Autodesk Inventor part; units mm, degrees
ref_plane "YZ Plane" through (0, 0, 0) normal (1, 0, 0) x (0, 1, 0)
ref_plane "XZ Plane" through (0, 0, 0) normal (0, 1, 0) x (-1, 0, 0)
ref_plane "XY Plane" through (0, 0, 0) normal (0, 0, 1) x (1, 0, 0)
sketch "草图1" plane through (0, 0, 0) normal (0, 0, 1) x (1, 0, 0)
  arc A0 (7.5, 0) -> (-7.5, 0) centre (0, 0) ccw
  arc A1 (15, 0) -> (-15, 0) centre (0, 0) ccw
  line L0 (25, 5) -> (25, 0)
  line L1 (-25, 0) -> (-25, 5)
  line L2 (25, 0) -> (7.5, 0)
  line L3 (-7.5, 0) -> (-25, 0)
  line L4 (-25, 5) -> (-5.5902, 5)
  line L5 (5.5902, 5) -> (25, 5)
  line L6 (0, 0) -> (0, -4.0409)
  line L7 (0, 0) -> (2.0046, 0)
  arc A2 (5.5902, 5) -> (-5.5902, 5) centre (0, 0) ccw
  arc A3 (14.1421, 5) -> (-14.1421, 5) centre (0, 0) ccw
  dimension "d0" = 15
  dimension "d1" = 30
  dimension "d2" = 5
  dimension "d3" = 50
  dimension "d4" = 4.0409
  dimension "d5" = 2.0046
extrude "拉伸1" add sketch "草图1" along normal blind 40
sketch "草图2" plane through (0, 0, 40) normal (0, 0, 1) x (1, 0, 0)
  line L0 (14.1421, 5) -> (25, 5)
  line L1 (25, 5) -> (14.1421, 5)
  line L2 (25, 5) -> (25, 0)
  line L3 (25, 0) -> (15, 0)
  line L4 (7.5, 0) -> (25, 0)
  line L5 (-14.1421, 5) -> (-25, 5)
  line L6 (-14.1421, 5) -> (-25, 5)
  line L7 (-25, 5) -> (-25, 0)
  line L8 (-25, 0) -> (-15, 0)
  arc A0 (15, 0) -> (14.1421, 5) centre (0, 0) ccw
  arc A1 (-14.1421, 5) -> (-15, 0) centre (0, 0) ccw
extrude "拉伸2" cut sketch "草图2" against normal blind 5
pattern_linear "矩形阵列1" count 2 spacing 35 along (0, 0, -1) of "拉伸2"
fillet "圆角1" radius 0.25 2 edges at (14.1421, 5, 20) (-14.1421, 5, 20)
sketch "草图3" plane through (25, 5, 35) normal (0, 1, 0) x (1, 0, 0)
  circle A0 centre (-5, 25) radius 2.5
  circle A1 centre (-5, 5) radius 2.5
  circle A2 centre (-45, 25) radius 2.5
  circle A3 centre (-45, 5) radius 2.5
  line L0 (0, 30) -> (0, 0)
  line L1 (0, 30) -> (-10.6822, 30)
  line L2 (-10.6822, 0) -> (0, 0)
  line L3 (-50, 30) -> (-50, 0)
  line L4 (-50, 0) -> (-39.3178, 0)
  line L5 (-39.3178, 30) -> (-50, 30)
  point P0 (-25, 35)
  dimension "d14" = 5
  dimension "d15" = 5
  dimension "d16" = 5
  dimension "d17" = 5
  dimension "d18" = 5
  dimension "d19" = 5
  dimension "d20" = 5
  dimension "d21" = 5
  dimension "d22" = 5
  dimension "d23" = 5
  dimension "d24" = 5
  dimension "d25" = 5
extrude "拉伸3" cut sketch "草图3" against normal through all
properties part number "砂轮架带动曲柄轴盖"
Can you work these out from the model? Positions are in its coordinate system, mm. A direction names the side the tool comes from. Round coordinates to 2 decimals unless told otherwise and drop trailing zeros. Write each loop counter-clockwise with the first axis right and the second up, starting at its lowest first coordinate (ties: lowest second). Pieces come first, ordered by that corner, then holes. Notation, with made-up numbers: M -9,22.5 L 34,22.5 A21 ccw 34,28.5 Z; hole C 84.5,-38.5 d8. An arc over 180 degrees is marked long. Use a Markdown table: item, result.
Item 1: Which directions (+Z, -Z, +X, -X, +Y, -Y) give clear straight access to the entire face, cutting with the end or side of a thin tool? Please do faces 1 (the face through (-14.78, 2.57, 2.54)), 2 (the face through (-20, 5, 20)), 3 (the face through (20, 5, 20)).
Found:
| item | result |
|---|---|
| face 1 | -Z, -X, +Y |
| face 2 | +Z, -Z, -X, +Y |
| face 3 | +Z, -Z, +X, +Y |
Item 2: We'd pull the mould along Z, two halves only. Please class faces 4 (the face through (25, 3, 20)), 5 (the face through (-20, 3, 5)), 6 (the face through (-21.84, 2.54, 28.31)): released by +Z, released by -Z, zero draft, split by the parting line, or undercut.
Found:
| item | result |
|---|---|
| face 4 | zero draft |
| face 5 | released by -Z |
| face 6 | undercut |
Item 3: For pin 1 Ø3 at (x, z) = (-17.5, 25.5) entering from +Y; pin 2 Ø4 at (x, z) = (-20, 10) entering from +Y; pin 3 Ø5.5 at (x, y) = (-21, 3) entering from +Z; pin 4 Ø8 at (x, z) = (-9.5, 22) entering from +Y, each with a flat end and sliding along its axis, tell me the tip position at first contact or that it passes through.
Found:
| item | result |
|---|---|
| pin 1 | stops at y = 5 |
| pin 2 | passes through |
| pin 3 | stops at z = 35 |
| pin 4 | stops at y = 13.96 |
Item 4: I want a section at D-D (z = 26). List the corners of the cut face in (x, y) for me.
Found:
| item | result |
|---|---|
| outline | M -25,0 L -7.5,0 A7.5 cw 7.5,0 L 25,0 L 25,5 L 14.32,5 A0.25 cw 14.08,5.16 A15 ccw -14.08,5.16 A0.25 cw -14.32,5 L -25,5 Z |
Item 5: I want a section at C-C (y = 6.5). List the corners of the cut face in (x, z) for me.
Found:
| item | result |
|---|---|
| outline | M -13.52,0 L -3.74,0 L -3.74,40 L -13.52,40 Z; M 3.74,0 L 13.52,0 L 13.52,40 L 3.74,40 Z |
Item 6: I want a section at B-B (z = 8.5). List the corners of the cut face in (x, y) for me.
Found:
| item | result |
|---|---|
| outline | M -25,0 L -22,0 L -22,5 L -25,5 Z; M -18,0 L -7.5,0 A7.5 cw 7.5,0 L 18,0 L 18,5 L 14.32,5 A0.25 cw 14.08,5.16 A15 ccw -14.08,5.16 A0.25 cw -14.32,5 L -18,5 Z; M 22,0 L 25,0 L 25,5 L 22,5 Z |
Item 7: I want a section at A-A (x = 20). List the corners of the cut face in (y, z) for me, and give its area (3 significant figures).
Found:
| item | result |
|---|---|
| outline | M 0,5 L 5,5 L 5,7.5 L 0,7.5 Z; M 0,12.5 L 5,12.5 L 5,27.5 L 0,27.5 Z; M 0,32.5 L 5,32.5 L 5,35 L 0,35 Z |
| area | 100 mm2 |
Item 8: If I drill on line 1 along Z through (x, y) = (-20, 1.85); line 2 along X through (y, z) = (4.5, 28.5); line 3 along X through (y, z) = (3.95, 30), over which ranges is the centre line in solid material (lowest first)? Write a range as [from, to].
Found:
| item | result |
|---|---|
| line 1 | z = [5, 7.5], [12.5, 27.5], [32.5, 35] |
| line 2 | x = [-25, -22], [-18, -6], [6, 18], [22, 25] |
| line 3 | x = [-25, -22.5], [-17.5, -6.38], [6.38, 17.5], [22.5, 25] |
